```python
from build123d import *

# Parameters (mm, degrees)
F1_W     = 18
F1_H     = 5
F1_R     = 1.25
F2_DEPTH = 1.5
F3_R     = 2
F4_R     = 0.5


with BuildPart() as f2:
    # F1 (on face) → F2 (new body)
    with BuildSketch(Plane.XY):
        with Locations((9, 2.5)):
            Rectangle(F1_W, F1_H)
        with Locations((15, 2.445588)):
            Circle(F1_R, mode=Mode.SUBTRACT)
        with Locations((3, 2.596398)):
            Circle(F1_R, mode=Mode.SUBTRACT)
    extrude(amount=F2_DEPTH)

    # F3
    f3_edges = [f2.edges().sort_by_distance(p)[0] for p in [
        (0, 5, 0.75),
        (0, 0, 0.75),
        (18, 0, 0.75),
        (18, 5, 0.75),
    ]]
    fillet(f3_edges, radius=F3_R)

    # F4
    f4_edges = [f2.edges().sort_by_distance(p)[0] for p in [
        (1.75, 2.596398, 1.5),
        (16.25, 2.445588, 0.75),
        (13.75, 2.445588, 0),
        (13.75, 2.445588, 1.5),
        (1.75, 2.596398, 0),
    ]]
    fillet(f4_edges, radius=F4_R)


solid = f2.part
```
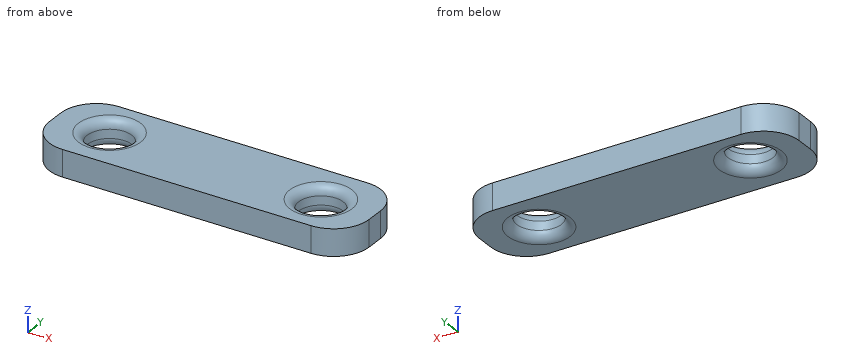
Design review of the part built by this model. Coordinates are the model's own, in mm. Coordinates: 2 decimals unless noted, no trailing zeros. Order: outer loops, then holes, each group sorted by start corner. A loop starts at its lowest first (then second) coordinate and runs counter-clockwise, first axis right, second up. Notation, with made-up numbers: (62.5, 62.5) - (70.5, 62.5) arc R25 ccw to (70.5, 99.5) - close; hole circle Ø9 at (87.5, 18). An arc over 180 degrees is marked (long way). Answer in a Markdown table with one row per item.
(1) Consider section A-A on x = 3. State the section outline as (y, z) points.
Checked values:
| item | result |
|---|---|
| outline | (0, 0) - (0.85, 0) arc R0.5 ccw to (1.35, 0.5) - (1.35, 1) arc R0.5 ccw to (0.85, 1.5) - (0, 1.5) - close; (3.85, 0.5) arc R0.5 ccw to (4.35, 0) - (5, 0) - (5, 1.5) - (4.35, 1.5) arc R0.5 ccw to (3.85, 1) - close |
(2) Clearance check with flat-ended pins moving along their axes: pin 1 (3 mm diameter, centred on x = 3, y = 2.6, fed in from +Z); pin 2 (3 mm diameter, centred on x = 15, y = 2.45, fed in from -Z). State where each tip first meets the part, or that it passes through.
Checked values:
| item | result |
|---|---|
| pin 1 | z = 1.44 |
| pin 2 | z = 0.06 |
(3) Consider section D-D on z = 0.3. State the section outline as (x, y) points, plus the area to 3 significant figures.
Checked values:
| item | result |
|---|---|
| outline | (0, 2) arc R2 ccw to (2, 0) - (16, 0) arc R2 ccw to (18, 2) - (18, 3) arc R2 ccw to (16, 5) - (2, 5) arc R2 ccw to (0, 3) - close; hole circle Ø2.58 at (3, 2.6); hole circle Ø2.58 at (15, 2.45) |
| area | 76.1 mm^2 |
(4) Consider section C-C on y = 3.25. Give the number of separate pieces and of enclosed holes in the cut face, plus the area to 3 significant figures.
Checked values:
| item | result |
|---|---|
| separate pieces | 3 |
| enclosed holes | 0 |
| area | 20.4 mm^2 |
(5) Consider section B-B on z = 1.25. State the section outline as (x, y) points, plus the area to 3 significant figures.
Checked values:
| item | result |
|---|---|
| outline | (0, 2) arc R2 ccw to (2, 0) - (16, 0) arc R2 ccw to (18, 2) - (18, 3) arc R2 ccw to (16, 5) - (2, 5) arc R2 ccw to (0, 3) - close; hole circle Ø2.63 at (3, 2.6); hole circle Ø2.63 at (15, 2.45) |
| area | 75.7 mm^2 |
(6) Wall thickness on line 1 along Y through (x, z) = (3, 0.7); line 2 along X through (y, z) = (3.35, 0.8); line 3 along X through (y, z) = (2.6, 1.4): over which ranges is each line inside the solid? List them lowest first. Write a range as from..to.
Checked values:
| item | result |
|---|---|
| line 1 | 0..1.35, 3.85..5 |
| line 2 | 0.03..2, 4..14.14, 15.86..17.97 |
| line 3 | 0..1.55, 4.45..13.56, 16.44..18 |
